from build123d import *

# Parameters (mm, degrees)
F0_W     = 10
F0_H     = 10
F1_DEPTH = 15
F2_SIZE  = 2
F3_R     = 2


with BuildPart() as f1:
    # F0 (on Front) → F1 (new body)
    with BuildSketch(Plane.XZ):
        with Locations((-5, 5)):
            Rectangle(F0_W, F0_H)
    extrude(amount=F1_DEPTH)

    # F2
    f2_edges = [f1.edges().sort_by_distance(p)[0] for p in [
        (-5, -15, 10),
        (0, -15, 5),
        (0, -7.5, 10),
    ]]
    chamfer(f2_edges, length=F2_SIZE)

    # F3
    f3_edges = [f1.edges().sort_by_distance(p)[0] for p in [
        (-10, 0, 5),
        (-6, 0, 10),
        (-10, -6.5, 10),
    ]]
    fillet(f3_edges, radius=F3_R)


solid = f1.part
Geometry: final body of the model. Coordinates: model frame, mm. Give positions to 0.01 mm unless a question says otherwise; leave off trailing zeros. Order: outer loops, then holes, each group sorted by start corner. A loop starts at its lowest first (then second) coordinate and runs counter-clockwise, first axis right, second up. Notation, with made-up numbers: (46.25, 86) - (98.25, 86) arc R18 ccw to (98.25, 116) - close; hole circle Ø3 at (19.5, -29.75). An arc over 180 degrees is marked (long way). Use CSV: the item, a comma, the result in double quotes.
1. Section query A-A (z = 3.25). Output: boundary loops of the cut face in (x, y).
Answers below:
outline,"(-10, -15) - (-2, -15) - (0, -13) - (0, 0) - (-8, 0) arc R2 ccw to (-10, -2) - close"
2. Section query B-B (y = -6.5). Output: boundary loops of the cut face in (x, z), plus the area to 3 significant figures.
Answers below:
outline,"(-10, 0) - (0, 0) - (0, 8) - (-2, 10) - (-8, 10) arc R2 ccw to (-10, 8) - close"
area,"97.1 mm2"
3. Material intervals for line 1 along Y through (x, z) = (-1.5, 5.75); line 2 along X through (y, z) = (-0.25, 6.75); line 3 along Z through (x, y) = (-6, -13.5), sorted ascending. Write a range as from..to.
Answers below:
line 1,"-14.5..0"
line 2,"-8.97..0"
line 3,"0..9.5"
